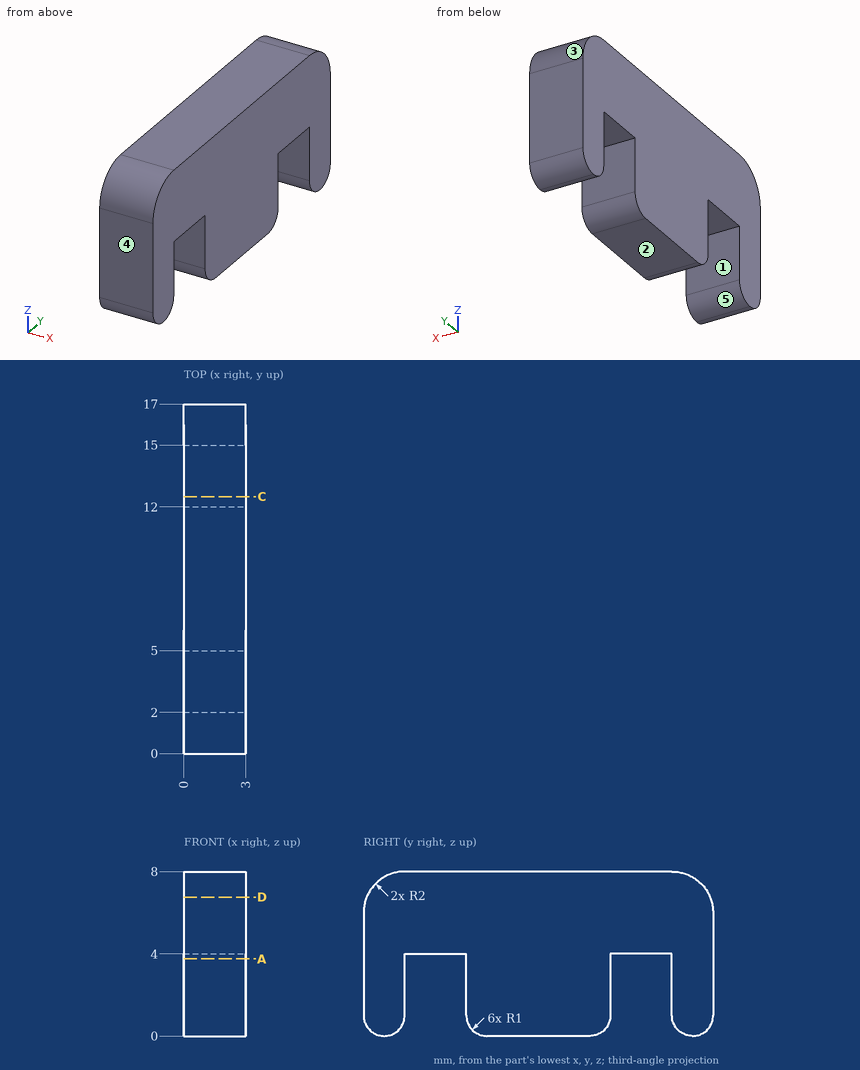
The drawing under review shows one solid part. Ordinate dimensions are in mm from its lowest x, y, z. A direction names the side the tool comes from. Coordinates: 2 decimals unless noted, no trailing zeros. Write each loop counter-clockwise with the first axis right and the second up, starting at its lowest first coordinate (ties: lowest second). Pieces come first, ordered by that corner, then holes. Notation, with made-up numbers: (-5.75, 84.25) - (20.25, 84.25) arc R21 ccw to (20.25, 119.25) - close; hole circle Ø5 at (-18.75, -30.75). An arc over 180 degrees is marked (long way). Answer in a Markdown table with one row per item. Add a question column.
Q1. Draft analysis for pull direction Y (two halves, no side actions). For the marked faces 3, 4 and 5, state which applies: +Y half, -Y half, draft (parallel to the pull), parting line (faces both ways), or undercut.
Q2. For probe 1 along Y at (x, z) = (2.5, 1); probe 2 along Z at (x, y) = (1.6, 13); probe 3 along Y at (x, z) = (0.85, 7.5) (1 decimal), list the stretches that pass through material, from the lowest coordinate up.
Q3. We need section D-D, the plane z = 6.75. State the section outline as (x, y) points (1 decimal).
Q4. For P1, Ø4, axis at y = 4, z = 1, coming from the +X side; P2, Ø1.5, axis at x = 1, y = 4, coming from the -Z side, all flat-tipped, find the tip position at first contact; note any pin that passes through.
Q5. We need section A-A, the plane z = 3.75. State the section outline as (x, y) points.
Q6. Tool access review of the marked faces 1 and 2: name each direction out of +Z, -Z, +X, -X, +Y, -Y from which nothing blocks a thin tool from reaching the whole face with its end or side.
Q7. We need section C-C, the plane y = 12.5. State the section outline as (x, z) points.
Answer list:
| question | item | result |
|---|---|---|
| 1 | face 3 | +Y half |
| 1 | face 4 | -Y half |
| 1 | face 5 | undercut |
| 2 | probe 1 | y = 0 to 2, 5 to 12, 15 to 17 |
| 2 | probe 2 | z = 4 to 8 |
| 2 | probe 3 | y = 0.7 to 16.3 |
| 3 | outline | (0, 0.1) - (3, 0.1) - (3, 16.9) - (0, 16.9) - close |
| 4 | P1 | stops at x = 3 |
| 4 | P2 | stops at z = 4 |
| 5 | outline | (0, 0) - (3, 0) - (3, 2) - (0, 2) - close; (0, 5) - (3, 5) - (3, 12) - (0, 12) - close; (0, 15) - (3, 15) - (3, 17) - (0, 17) - close |
| 6 | face 1 | -Z, +X, -X |
| 6 | face 2 | -Z, +X, -X, +Y, -Y |
| 7 | outline | (0, 4) - (3, 4) - (3, 8) - (0, 8) - close |
